Autodesk Inventor part; units mm, degrees
ref_plane "YZ Plane" through (0, 0, 0) normal (1, 0, 0) x (0, 1, 0)
ref_plane "XZ Plane" through (0, 0, 0) normal (0, 1, 0) x (-1, 0, 0)
ref_plane "XY Plane" through (0, 0, 0) normal (0, 0, 1) x (1, 0, 0)
sketch "草圖1" plane through (0, 0, 0) normal (0, 1, 0) x (-1, 0, 0)
  circle A0 centre (0, 0) radius 3.5
  line L0 (10, 20) -> (-10, 20)
  line L1 (-10, 20) -> (-10, -20)
  line L2 (-10, -20) -> (10, -20)
  line L3 (10, -20) -> (10, 20)
  line L4 (10, 20) -> (-10, -20) construction
  line L5 (-10, 20) -> (10, -20) construction
  line L6 (-95, 0) -> (-95, 5)
  line L7 (-95, 5) -> (-95, -5)
  line L8 (-95, -5) -> (-110, -5)
  line L9 (-110, -5) -> (-110, -10)
  line L10 (-110, -10) -> (-10, -20)
  line L11 (-95, -5) -> (-95, 5)
  line L12 (-95, 5) -> (-110, 5)
  line L13 (-110, 5) -> (-110, 10)
  line L14 (-110, 10) -> (-10, 20)
  dimension "d0" = 7
  dimension "d1" = 20
  dimension "d2" = 40
  dimension "d8" = 20
  dimension "d9" = 10
  dimension "d10" = 120
  dimension "d11" = 15
extrude "擠出1" add sketch "草圖1" along normal blind 5
sketch "草圖2" plane through (-10, 0, 20) normal (0, 0, 1) x (1, 0, 0)
  line L0 (20, 0) -> (120, 0)
  line L1 (120, 0) -> (114, 0)
  line L2 (114, 0) -> (114, 2.5)
  circle A0 centre (114, 2.5) radius 1.5
  point P0 (10, 0)
  dimension "d14" = 6
  dimension "d15" = 2.5
  dimension "d16" = 3
extrude "擠出2" cut sketch "草圖2" against normal through all
properties part number "4. 托板"
Input: part model. Units: mm. Frame: model coordinates. A direction names the side the tool comes from. Coordinates: 2 decimals unless noted, no trailing zeros. Write each loop counter-clockwise with the first axis right and the second up, starting at its lowest first coordinate (ties: lowest second). Pieces come first, ordered by that corner, then holes. Notation, with made-up numbers: M -23.75,73.5 L 10.25,73.5 A21 cw 10.25,103.5 Z; hole C -34.75,-34.75 d10. An arc over 180 degrees is marked long. Answer as a JSON object with one key per item and string values. Group by question number.
(1) Mould query, pull axis X, two halves, no side actions, for faces 3 (the face through (102.8, 1.6, -7.8)), 4 (the face through (102.5, 2.57, 7.92)), 5 (the face through (102, 2, 5)), 6 (the face through (110, 2, -7)). Classes: pulls with the +X half, pulls with the -X half, needs draft (parallel to the pull), parting line crosses it, or undercut.
(2) Contact query for flat-ended pins moving along their axis: P1, Ø1.5, axis at x = 101.5, y = 1.5, coming from the -Z side (3 decimals); P2, Ø1, axis at y = 1, z = 2, coming from the +X side; P3, Ø3, axis at x = 21.5, y = 3, coming from the -Z side. Output: stop coordinate, or through.
(3) Ray query, line 1 along X through (y, z) = (2.5, -9.3); line 2 along Z through (x, y) = (0, 1.1); line 3 along Y through (x, z) = (104, -7.2). Return the intervals inside material, ascending. Write a range as [from, to].
(4) Section A-A on y = 2.5. Output: boundary loops of the cut face in (x, z), plus the area to 3 significant figures.
(5) Set-up query: faces 1 (the face through (95, 2, 0)), 2 (the face through (0, 2, 20)). Return all of +Z, -Z, +X, -X, +Y, -Y with unobstructed straight access to the full face (end or side cutting, diameter ignored); none if empty.
(6) Section C-C on x = 104. Output: boundary loops of the cut face in (y, z).
(7) Section D-D on x = 0. Output: boundary loops of the cut face in (y, z).
(8) Section B-B on z = 0. Output: boundary loops of the cut face in (x, y).
Result set:
{
 "1": {"face 3": "undercut", "face 4": "undercut", "face 5": "needs draft", "face 6": "pulls with the +X half"},
 "2": {"P1": "stops at z = -10.925", "P2": "stops at x = 95", "P3": "stops at z = -19"},
 "3": {"line 1": "x = [-10, 102.5], [105.5, 110]", "line 2": "z = [-20, -3.5], [3.5, 20]", "line 3": "y = [0, 1], [4, 5]"},
 "4": {"outline": "M -10,-20 L 10,-20 L 102.5,-10.75 L 102.5,-5 L 95,-5 L 95,5 L 102.5,5 L 102.5,10.75 L 10,20 L -10,20 Z; M 105.5,-10.45 L 110,-10 L 110,-5 L 105.5,-5 Z; M 105.5,5 L 110,5 L 110,10 L 105.5,10.45 Z; hole C 0,0 d7", "area": "3,580 mm2"},
 "5": {"face 1": "+X, +Y, -Y", "face 2": "+Z, +X, -X, +Y, -Y"},
 "6": {"outline": "M 0,-10.6 L 1,-10.6 L 1,-5 L 0,-5 Z; M 0,5 L 1,5 L 1,10.6 L 0,10.6 Z; M 4,-10.6 L 5,-10.6 L 5,-5 L 4,-5 Z; M 4,5 L 5,5 L 5,10.6 L 4,10.6 Z"},
 "7": {"outline": "M 0,-20 L 5,-20 L 5,-3.5 L 0,-3.5 Z; M 0,3.5 L 5,3.5 L 5,20 L 0,20 Z"},
 "8": {"outline": "M -10,0 L -3.5,0 L -3.5,5 L -10,5 Z; M 3.5,0 L 95,0 L 95,5 L 3.5,5 Z"}
}
